The listing builds one solid part. Answer for the finished solid, in the listing's coordinates (mm). A direction names the side the tool comes from. Round coordinates to 2 decimals unless told otherwise and drop trailing zeros. Write each loop counter-clockwise with the first axis right and the second up, starting at its lowest first coordinate (ties: lowest second). Pieces come first, ordered by that corner, then holes. Notation, with made-up numbers: (39, -35.5) - (73, -35.5) arc R22 cw to (73, -25.5) - close; hole circle Ø7 at (36, -33.75). An arc over 180 degrees is marked (long way). Answer as CSV lines item,"result". Start each with the question number.
Item 1: Which of the six approach directions +Z, -Z, +X, -X, +Y, -Y give full straight-line access (tool end or side, diameter ignored) to faces 1 (the cylindrical face through (-0.1, 8.2, 2.9)), 2 (the cylindrical face through (-0.54, 5.06, 2.44))?
Item 2: A cutting plane is placed at B-B on y = 11.75. Determine the outline of the cut face in (x, z) (3 decimals).
Item 3: A cutting plane is placed at A-A on y = 17. Determine the outline of the cut face in (x, z) (3 decimals), and give its area (3 significant figures).
Item 4: A cutting plane is placed at C-C on z = 0. Determine the outline of the cut face in (x, y).
Item 5: Straight lines are drawn through the part: line 1 along Z through (x, y) = (0.2, 11) (3 decimals); line 2 along Y through (x, z) = (2.65, 0); line 3 along X through (y, z) = (15.25, -2.2). For each, find the intervals that lie inside material, in ascending order. Write a range as [from, to].
Item 6: A cutting plane is placed at D-D on x = 1.65. Determine the outline of the cut face in (y, z), and give its area (3 significant figures).
Item 7: Flat-ended cylindrical pins translate along their axes: pin 1 (0.8 mm diameter, centred on x = 0, z = 2, fed in from +Y); pin 2 (0.8 mm diameter, centred on y = 11, z = -2, fed in from -X); pin 3 (0.6 mm diameter, centred on y = 12.5, z = -2, fed in from +X); pin 4 (1 mm diameter, centred on x = 0, y = 9, fed in from -Z). Find the tip coordinate at first contact, or state that the pin passes through.
```python
from build123d import *

# Parameters (mm, degrees)
ENL_V_MAT_EXTRU_1_REACH = 10.724
ESQUISSE3_W             = 0.7
ESQUISSE3_H             = 0.7
BOSS_EXTRU_1_DEPTH      = 10
ENL_V_START             = -3.25
ENL_V_MAT_EXTRU_2_DEPTH = 5.8


with BuildPart() as part:
    # Esquisse1 → Révolution1 (revolve)
    with BuildSketch(Plane.XY):
        with BuildLine():
            Line((2.5, 7.7), (2.5, 2.5))
            ThreePointArc((2.5, 2.5), (1.767766953, 0.732233047), (0, 0))
            Line((0, 0), (0, 8.7))
            Line((0, 8.7), (2.9, 8.7))
            Line((2.9, 8.7), (2.9, 7.7))
            Line((2.9, 7.7), (2.5, 7.7))
        make_face()
    revolve(axis=Axis((0, 0, 0), (0, 1, 0)))

    # Esquisse2 → Enlèv. mat.-Extru.1 (cut, up to next)
    with BuildSketch(Plane(origin=(0, 7.7, 0), x_dir=(-1, 0, 0), z_dir=(0, -1, 0)), mode=Mode.PRIVATE) as enl_v_mat_extru_1_sk1:
        Polygon((2.031643218, 2.5), (-2.119175806, 2.5), (-0.304277426, 5.41579693), align=None)
    enl_v_mat_extru_1_tool1 = extrude(enl_v_mat_extru_1_sk1.sketch, amount=-ENL_V_MAT_EXTRU_1_REACH, mode=Mode.PRIVATE) & part.part
    add(enl_v_mat_extru_1_tool1.solids().sort_by_distance((0.130603, 7.7, -3.471932))[0], mode=Mode.SUBTRACT)

    # Esquisse3 → Boss.-Extru.1 (add)
    with BuildSketch(Plane(origin=(0, 8.7, 0), x_dir=(1, 0, 0), z_dir=(0, 1, 0))):
        with Locations((0, 1.905)):
            Rectangle(ESQUISSE3_W, ESQUISSE3_H)
        with Locations((0, -0.635)):
            Rectangle(ESQUISSE3_W, ESQUISSE3_H)
        with Locations((0, -1.905)):
            Rectangle(ESQUISSE3_W, ESQUISSE3_H)
        with Locations((0, 0.635)):
            Rectangle(ESQUISSE3_W, ESQUISSE3_H)
    extrude(amount=BOSS_EXTRU_1_DEPTH)

    # Esquisse4 → Enlèv. mat.-Extru.2 (cut)
    with BuildSketch(Plane.ZY.offset(0.35).offset(ENL_V_START)):
        Polygon((-2.885095567, 16.2), (-1.265657514, 16.2), (-1.265657514, 33.921907916), (0, 33.921907916), (0, 17.43), (1.344412991, 17.43), (1.344412991, 16.2), (2.897512796, 16.2), (2.897512796, 34.676886987), (-2.885095567, 34.676886987), align=None)
    extrude(amount=ENL_V_MAT_EXTRU_2_DEPTH, mode=Mode.SUBTRACT)


solid = part.part
```
Geometry says:
1,face 1,"+Y, -Y"
1,face 2,"-Y"
2,outline,"(-0.35, -2.255) - (0.35, -2.255) - (0.35, -1.555) - (-0.35, -1.555) - close; (-0.35, -0.985) - (0.35, -0.985) - (0.35, -0.285) - (-0.35, -0.285) - close; (-0.35, 0.285) - (0.35, 0.285) - (0.35, 0.985) - (-0.35, 0.985) - close; (-0.35, 1.555) - (0.35, 1.555) - (0.35, 2.255) - (-0.35, 2.255) - close"
3,outline,"(-0.35, -0.985) - (0.35, -0.985) - (0.35, -0.285) - (-0.35, -0.285) - close; (-0.35, 0.285) - (0.35, 0.285) - (0.35, 0.985) - (-0.35, 0.985) - close"
3,area,"0.980 mm^2"
4,outline,"(-2.9, 7.7) - (-2.5, 7.7) - (-2.5, 2.5) arc R2.5 ccw to (2.5, 2.5) - (2.5, 7.7) - (2.9, 7.7) - (2.9, 8.7) - (-2.9, 8.7) - close"
5,line 1,"z = [-2.255, -1.555], [-0.985, -0.285], [0.285, 0.985], [1.555, 2.255]"
5,line 2,"y = [7.7, 8.7]"
5,line 3,"x = [-0.35, 0.35]"
6,outline,"(2.5, -1.88) - (7.7, -1.88) - (7.7, -2.38) - (8.7, -2.38) - (8.7, 2.38) - (7.7, 2.38) - (7.7, 1.88) - (2.5, 1.88) arc R1.88 ccw to start"
6,area,"29.8 mm^2"
7,pin 1,"stops at y = 16.2"
7,pin 2,"stops at x = -0.35"
7,pin 3,"stops at x = 0.35"
7,pin 4,"stops at z = -2.5"
